The model under review builds one solid part; all positions refer to its coordinate system, in mm. A direction names the side the tool comes from. Round coordinates to 2 decimals unless told otherwise and drop trailing zeros. Order: outer loops, then holes, each group sorted by start corner. A loop starts at its lowest first (then second) coordinate and runs counter-clockwise, first axis right, second up. Notation, with made-up numbers: M 28,52.25 L 51,52.25 A15 ccw 51,67.25 Z; hole C 39.25,-6.5 d7. An arc over 180 degrees is marked long. Answer as a JSON object with one key per item and string values. Group by question number.
1. Mouldability with a two-part tool opening along X and no side actions: class faces 4 (the face through (0, 6, 2.901)), 5 (the face through (0, -19, -15)), 6 (the face through (0, -7, 4.901)), 7 (the face through (-4.225, -2.544, 2.485)) as released by +X, released by -X, zero draft, split by the parting line, or undercut.
2. Add section D-D on x = 4.5. State the section outline as (y, z) points.
3. Machinability: for faces 1 (the face through (4.225, -2.544, -2.485)), 2 (the face through (-2.5, 5.92, -1.47)), 3 (the face through (0, -3, -4.901)), which of the approach directions +Z, -Z, +X, -X, +Y, -Y give a long, thin tool a straight path to every point of the face, cutting with its end or side? Answer none if there is none.
4. Add section C-C on z = -1.5. State the section outline as (x, y) points.
5. To check wall thickness, follow probe 1 along Y at (x, z) = (12, -1.5); probe 2 along Z at (x, y) = (1, -14); probe 3 along Z at (x, y) = (-3, 2). State the ranges of each line that lie inside material, in increasing order. Write a range as [from, to].
6. Add section A-A on x = 0. State the section outline as (y, z) points.
7. Add section B-B on y = -11.5. State the section outline as (x, z) points, and give its area (3 significant figures).
8. Clearance check with flat-ended pins moving along their axes: P1, Ø8, axis at y = -8, z = -9.5, coming from the -X side; P2, Ø1.5, axis at y = 7, z = -0.5, coming from the -X side; P3, Ø3, axis at x = 0, y = -8, coming from the -Z side; P4, Ø3, axis at y = -1, z = -4.5, coming from the +X side. State where each tip first meets the part, or that it passes through.
```python
from build123d import *

# Parameters (mm, degrees)
BOSS_EXTRUDE1_DEPTH = 12
BOSS_EXTRUDE2_DEPTH = 17.5
BOSS_EXTRUDE3_DEPTH = 2.5


with BuildPart() as part:
    # Sketch1 → Boss-Extrude1 (new body)
    with BuildSketch(Plane(origin=(0, 0, 0), x_dir=(1, 0, 0), z_dir=(0, 1, 0))):
        Polygon((-2.829700538, 4.901185103), (-5.659401077, 0), (-2.829700538, -4.901185103), (2.829700538, -4.901185103), (5.659401077, 0), (2.829700538, 4.901185103), align=None)
        Polygon((-1.675, 2.901185103), (-3.35, 0), (-1.675, -2.901185103), (1.675, -2.901185103), (3.35, 0), (1.675, 2.901185103), align=None, mode=Mode.SUBTRACT)
    extrude(amount=BOSS_EXTRUDE1_DEPTH)

    # Sketch2 → Boss-Extrude2 (add)
    with BuildSketch(Plane.XZ):
        Polygon((-2.829700538, -4.901185103), (2.829700538, -4.901185103), (5.659401077, 0), (2.829700538, 4.901185103), (-2.829700538, 4.901185103), (-5.659401077, 0), align=None)
    extrude(amount=BOSS_EXTRUDE2_DEPTH)

    # Sketch3 → Boss-Extrude3 (add)
    with BuildSketch(Plane.XZ.offset(17.5)):
        with BuildLine():
            Line((-14.176684542, 4.901185103), (14.176684542, 4.901185103))
            ThreePointArc((14.176684542, 4.901185103), (0, -15), (-14.176684542, 4.901185103))
        make_face()
    extrude(amount=BOSS_EXTRUDE3_DEPTH)


solid = part.part
```
Recorded:
{
 "1": {"face 4": "undercut", "face 5": "split by the parting line", "face 6": "zero draft", "face 7": "released by -X"},
 "2": {"outline": "M -20,-14.31 L -17.5,-14.31 L -17.5,-2.01 L 12,-2.01 L 12,2.01 L -17.5,2.01 L -17.5,4.9 L -20,4.9 Z"},
 "3": {"face 1": "-Z, +X, +Y", "face 2": "+Y", "face 3": "-Z, +X, -X, +Y"},
 "4": {"outline": "M -14.92,-20 L 14.92,-20 L 14.92,-17.5 L 4.79,-17.5 L 4.79,12 L 2.48,12 L 2.48,0 L -2.48,0 L -2.48,12 L -4.79,12 L -4.79,-17.5 L -14.92,-17.5 Z"},
 "5": {"probe 1": "y = [-20, -17.5]", "probe 2": "z = [-4.9, 4.9]", "probe 3": "z = [-4.61, -0.61], [0.61, 4.61]"},
 "6": {"outline": "M -20,-15 L -17.5,-15 L -17.5,-4.9 L 12,-4.9 L 12,-2.9 L 0,-2.9 L 0,2.9 L 12,2.9 L 12,4.9 L -20,4.9 Z"},
 "7": {"outline": "M -5.66,0 L -2.83,-4.9 L 2.83,-4.9 L 5.66,0 L 2.83,4.9 L -2.83,4.9 Z", "area": "83.2 mm²"},
 "8": {"P1": "passes through", "P2": "stops at x = -5.66", "P3": "stops at z = -4.9", "P4": "stops at x = 3.93"}
}
